Check sheet for the modelled part. Datum: model origin and axes. Units: mm. Coordinates: 2 decimals unless noted, no trailing zeros. Loops run counter-clockwise (first coordinate to the right, second up) from the corner with the lowest first, then second, coordinate; pieces in that order, holes last. Notation, with made-up numbers: (8, -33.5) - (63, -33.5) arc R8 ccw to (63, -22.5) - close; hole circle Ø11 at (17.5, 44.25). An arc over 180 degrees is marked (long way). Write each question's results on one line, items separated by ' | '. Start each with the question number.
1. Cross-section at D-D (x = 85.5). Record the cut outline in (y, z), and give its area (3 significant figures).
2. Gauge pin test, flat ends, axial feed: P1, Ø2, axis at x = 15.5, y = 2, coming from the +Z side; P2, Ø2, axis at y = 2.5, z = 65.5, coming from the -X side. Record the tip position at first contact, or that the pin passes through.
3. Cross-section at B-B (y = 4). Give the number of separate pieces and of enclosed holes in the cut face, and give its area (3 significant figures).
4. Cross-section at C-C (z = 76.5). Record the cut outline in (x, y).
5. Thickness scan on line 1 (X direction, y = 3.2, z = -149.5); line 2 (X direction, y = 1.85, z = -75); line 3 (X direction, y = 1.15, z = -102). Record the ranges inside material, lowest first. Write a range as [from, to].
6. Cross-section at A-A (x = -16.5). Record the cut outline in (y, z).
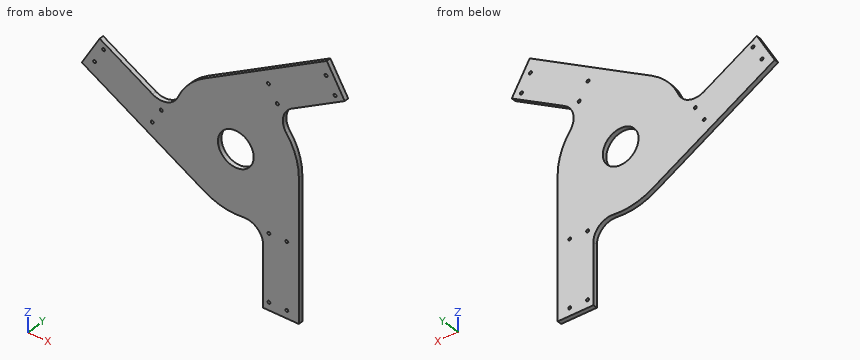
```python
from build123d import *

# Parameters (mm, degrees)
SKETCH_2_R          = 70.51
EXTRUDE_1_DEPTH     = 5
SKETCH_3_R          = 20
CUT_EXTRUDE_1_DEPTH = 235.001208449
HOLE_WIZARD_M4_1_D  = 3.3


with BuildPart() as part:
    # 스케치2 → 보스-돌출1 (new body)
    with BuildSketch(Plane(origin=(0, 0, 0), x_dir=(1, 0, 0), z_dir=(0, 1, 0))):
        with BuildLine():
            ThreePointArc((-70.305885551, -5.361208523), (-62.360516315, 32.906323175), (-35.255, 61.063451221))
            Line((-35.255, 61.063451221), (-172.303520149, -18.061548779))
            Line((-172.303520149, -18.061548779), (-152.303520149, -52.702564931))
            Line((-152.303520149, -52.702564931), (-93.108708968, -18.52642476))
            Line((-93.108708968, -18.52642476), (-70.305885551, -5.361208523))
        make_face()
        with BuildLine():
            ThreePointArc((-64.74417268, -27.925833988), (-68.461084842, -16.874239606), (-70.305885551, -5.361208523))
            Line((-70.305885551, -5.361208523), (-93.108708968, -18.52642476))
            ThreePointArc((-93.108708968, -18.52642476), (-76.817557222, -16.862165002), (-64.74417268, -27.925833988))
        make_face()
        Circle(SKETCH_2_R)
        with BuildLine():
            Line((62.598708968, -71.371294899), (39.795885551, -58.206078662))
            ThreePointArc((39.795885551, -58.206078662), (2.682546343, -70.45895291), (-35.255, -61.063451221))
            Line((-35.255, -61.063451221), (101.793520149, -140.188451221))
            Line((101.793520149, -140.188451221), (121.793520149, -105.547435069))
            Line((121.793520149, -105.547435069), (62.598708968, -71.371294899))
        make_face()
        with BuildLine():
            ThreePointArc((62.598708968, -71.371294899), (53.011841866, -58.09487351), (56.556567996, -42.107181294))
            ThreePointArc((56.556567996, -42.107181294), (48.84406259, -50.85191884), (39.795885551, -58.206078662))
            Line((39.795885551, -58.206078662), (62.598708968, -71.371294899))
        make_face()
        with BuildLine():
            Line((30.51, 89.89771966), (30.51, 63.567287185))
            ThreePointArc((30.51, 63.567287185), (59.677969972, 37.552629735), (70.51, 0))
            Line((70.51, 0), (70.51, 158.25))
            Line((70.51, 158.25), (30.51, 158.25))
            Line((30.51, 158.25), (30.51, 89.89771966))
        make_face()
        with BuildLine():
            ThreePointArc((8.187604685, 70.033015282), (19.617022252, 67.726158447), (30.51, 63.567287185))
            Line((30.51, 63.567287185), (30.51, 89.89771966))
            ThreePointArc((30.51, 89.89771966), (23.805715357, 74.957038512), (8.187604685, 70.033015282))
        make_face()
    extrude(amount=EXTRUDE_1_DEPTH)

    # 스케치3 → 컷-돌출1 (cut, through all)
    with BuildSketch(Plane(origin=(0, 5, 0), x_dir=(1, 0, 0), z_dir=(0, 1, 0))):
        with Locations(Location((0, 0, 0), (0, 0, 270))):
            Circle(SKETCH_3_R)
    extrude(amount=-CUT_EXTRUDE_1_DEPTH, mode=Mode.SUBTRACT)

    # M4 나사 구멍1 (through all)
    with Locations(Plane(origin=(0, 5, 0), x_dir=(1, 0, 0), z_dir=(0, 1, 0))):
        with Locations((57.01, 149.5), (37.01, 75), (37.01, 149.5), (57.01, 75), (100.965797866, -124.12210827), (46.446905284, -69.551600194), (110.965797866, -106.801600194), (36.446905284, -86.87210827), (-157.975797866, -25.37789173), (-83.456905284, -5.448399806), (-147.975797866, -42.698399806), (-93.456905284, 11.87210827)):
            Hole(HOLE_WIZARD_M4_1_D / 2)


solid = part.part
```
Established:
1) outline: (0, 84.59) - (5, 84.59) - (5, 130.78) - (0, 130.78) - close | area: 231 mm^2
2) P1: z = 90.94 | P2: x = -29.3
3) separate pieces: 1 | enclosed holes: 13 | area: 28,200 mm^2
4) outline: (-8.52, 0) - (71.48, 0) - (71.48, 5) - (-8.52, 5) - close
5) line 1: [30.51, 35.36], [38.66, 55.36], [58.66, 70.51] | line 2: [23.85, 35.36], [38.66, 55.36], [58.66, 70.51] | line 3: [30.51, 70.51]
6) outline: (0, -68.55) - (5, -68.55) - (5, -11.3) - (0, -11.3) - close; (0, 11.3) - (5, 11.3) - (5, 71.89) - (0, 71.89) - close
